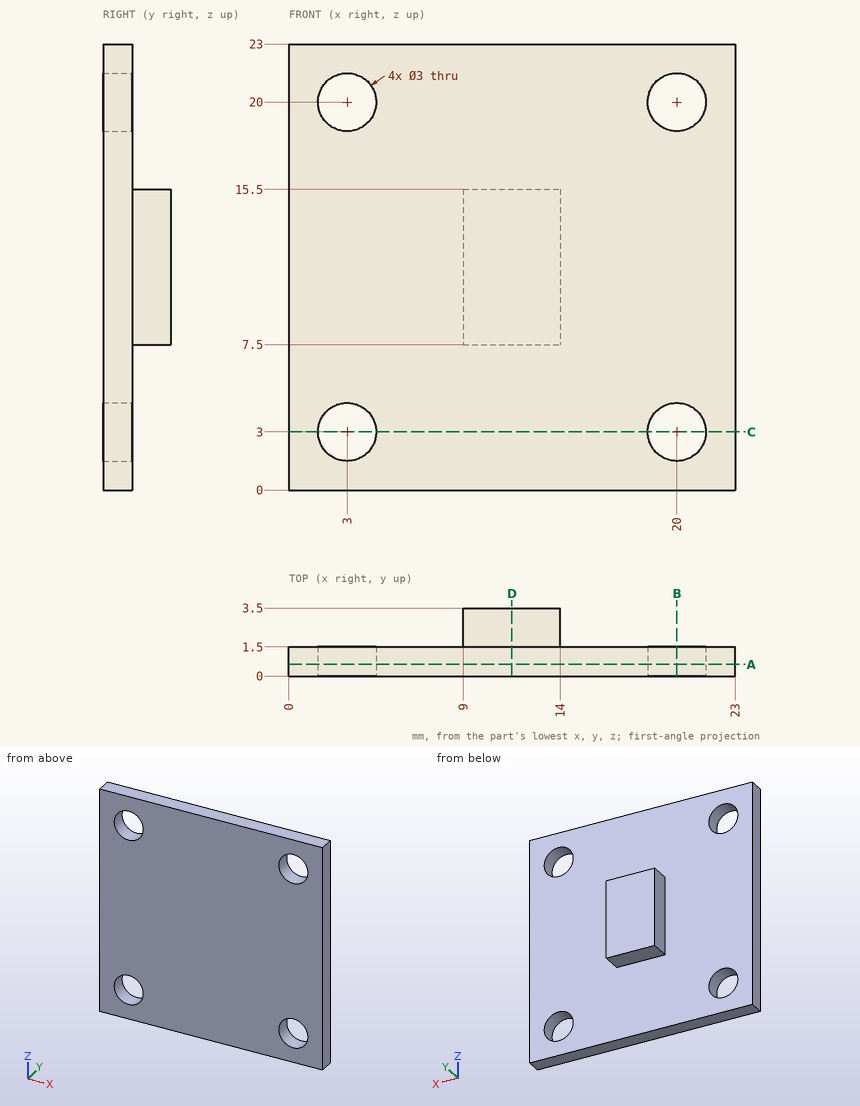
Could you check a few things on this drawing? It's one solid part, dimensions in mm from its lowest x, y, z. Give positions to 0.01 mm unless a question says otherwise; leave off trailing zeros. Write each loop counter-clockwise with the first axis right and the second up, starting at its lowest first coordinate (ties: lowest second). Pieces come first, ordered by that corner, then holes. Notation, with made-up numbers: M -6,78 L 51,78 A21 cw 51,90 Z; hole C 65.5,66 d1. An arc over 180 degrees is marked long. Put each result on its own line as item: value. Start each with the question number.
Item 1: I need wall thicknesses on L1, parallel to X at y = 0.3, z = 20; L2, parallel to X at y = 0.5, z = 21; L3, parallel to Y at x = 5.5, z = 2.75. Which ranges of each line are inside material? Lowest first, please. Write a range as from..to.
Item 2: If we section it at D-D, the plane x = 11.5: Write out the boundary of the cut face in (y, z).
Item 3: Will these pins go through, and if not, where does the flat tip stop? pin 1 (2 mm diameter, centred on x = 10.5, y = 3, fed in from -Z); pin 2 (2.5 mm diameter, centred on x = 20, z = 20, fed in from +Y); pin 3 (2 mm diameter, centred on y = 3, z = 11, fed in from +X).
Item 4: If we section it at C-C, the plane z = 3: Write out the boundary of the cut face in (x, y), then the cut area to 3 significant figures.
Item 5: If we section it at A-A, the plane y = 0.6: Write out the boundary of the cut face in (x, z), then the cut area to 3 significant figures.
Item 6: If we section it at B-B, the plane x = 20: Write out the boundary of the cut face in (y, z).
Values:
1. L1: 0..1.5, 4.5..18.5, 21.5..23
1. L2: 0..1.88, 4.12..18.88, 21.12..23
1. L3: 0..1.5
2. outline: M 0,0 L 1.5,0 L 1.5,7.5 L 3.5,7.5 L 3.5,15.5 L 1.5,15.5 L 1.5,23 L 0,23 Z
3. pin 1: z = 7.5
3. pin 2: through
3. pin 3: x = 14
4. outline: M 0,0 L 1.5,0 L 1.5,1.5 L 0,1.5 Z; M 4.5,0 L 18.5,0 L 18.5,1.5 L 4.5,1.5 Z; M 21.5,0 L 23,0 L 23,1.5 L 21.5,1.5 Z
4. area: 25.5 mm²
5. outline: M 0,0 L 23,0 L 23,23 L 0,23 Z; hole C 3,3 d3; hole C 3,20 d3; hole C 20,3 d3; hole C 20,20 d3
5. area: 501 mm²
6. outline: M 0,0 L 1.5,0 L 1.5,1.5 L 0,1.5 Z; M 0,4.5 L 1.5,4.5 L 1.5,18.5 L 0,18.5 Z; M 0,21.5 L 1.5,21.5 L 1.5,23 L 0,23 Z
